The model under review builds one solid part; all positions refer to its coordinate system, in mm. A direction names the side the tool comes from. Coordinates: 2 decimals unless noted, no trailing zeros. Write each loop counter-clockwise with the first axis right and the second up, starting at its lowest first coordinate (ties: lowest second). Pieces come first, ordered by that corner, then holes. Notation, with made-up numbers: (3, -19.75) - (36, -19.75) arc R19 cw to (36, -7.75) - close; hole circle Ø1 at (46.25, 59.5). An arc over 180 degrees is marked (long way). Return JSON: item names as keys, results as strings. Group by question number.
(1) We need section C-C on z = 7.5. State the section outline as (x, y) points (3 decimals).
(2) For pin 1 Ø1.5 at (x, z) = (-7, -12.5) entering from -Y; pin 2 Ø2 at (x, y) = (-4.5, 6) entering from +Z; pin 3 Ø4.5 at (x, z) = (-1.5, 4.5) entering from +Y (3 decimals); pin 4 Ø5 at (y, z) = (-6.5, -3.5) entering from +X, all flat-tipped, find the tip position at first contact; note any pin that passes through.
(3) To check wall thickness, follow L1, parallel to Y at x = 0, z = -8.25 (3 decimals); L2, parallel to Y at x = 1.75, z = -2; L3, parallel to X at y = -4, z = 5 (3 decimals). State the ranges of each line that lie inside material, in increasing order. Write a range as from..to.
(4) Tool access review of faces 1 (the face through (10.045, 0, 7)), 2 (the face through (1, 10.06, 7)), 3 (the face through (6, 0, -25)), 4 (the face through (5.2, 1.4, -0.48)): name each direction out of +Z, -Z, +X, -X, +Y, -Y from which nothing blocks a thin tool from reaching the whole face with its end or side.
(5) We need section A-A on y = 0. State the section outline as (x, z) points (3 decimals), then the cut area to 3 significant figures.
(6) We need section D-D on z = -18. State the section outline as (x, y) points (3 decimals).
(7) Draft analysis for pull direction Y (two halves, no side actions). For faces 5 (the face through (-7, -2, 15)), 6 (the face through (-10.4, -7.974, -5.28)), 7 (the face through (1, -7.46, 7)), state which applies: released by +Y, released by -Y, zero draft, split by the parting line, or undercut.
(8) We need section B-B on x = 0. State the section outline as (y, z) points (3 decimals), then the cut area to 3 significant figures.
```python
from build123d import *

# Parameters (mm, degrees)
F1_R          = 13.105
F1_R_2        = 5
F2_DEPTH      = 25
F2_DEPTH_BACK = 15
F5_DEPTH      = 15.48


with BuildPart() as f2:
    # F1 (on Top) → F2 (new body, two sides)
    with BuildSketch(Plane.XY) as f2_sk:
        Circle(F1_R)
        Circle(F1_R_2, mode=Mode.SUBTRACT)
    extrude(amount=-F2_DEPTH)
    extrude(f2_sk.sketch, amount=F2_DEPTH_BACK)

    # F4 (on offset) → F5 (cut)
    with BuildSketch(Plane.XY.offset(15)):
        Polygon((10.0449961981, 10.0600004722), (-6.8450038019, 10.0600004722), (-6.8450038019, -5.8399995278), (-6.8450038019, -7.4599995278), (10.0449961981, -7.4599995278), align=None)
    extrude(amount=-F5_DEPTH, mode=Mode.SUBTRACT)


solid = f2.part
```
Ans:
{
 "1": {"outline": "(-6.845, -7.46) - (-6.845, 10.06) - (8.399, 10.06) arc R13.105 ccw (long way) to (10.045, 8.417) - (10.045, -7.46) - close"},
 "2": {"pin 1": "y = -11.52", "pin 2": "z = -0.48", "pin 3": "y = 13.105", "pin 4": "x = 12.48"},
 "3": {"L1": "-13.105..-5, 5..13.105", "L2": "-12.99..-4.68, 4.68..12.99", "L3": "-12.48..-6.845, 10.045..12.48"},
 "4": {"face 1": "+Z, +Y", "face 2": "+Z, +X", "face 3": "-Z, +X, -X, +Y, -Y", "face 4": "+Z"},
 "5": {"outline": "(-13.105, -25) - (-5, -25) - (-5, -0.48) - (-6.845, -0.48) - (-6.845, 15) - (-13.105, 15) - close; (5, -25) - (13.105, -25) - (13.105, 15) - (10.045, 15) - (10.045, -0.48) - (5, -0.48) - close", "area": "542 mm²"},
 "6": {"outline": "circle Ø26.21 at (0, 0); hole circle Ø10 at (0, 0)"},
 "7": {"face 5": "zero draft", "face 6": "split by the parting line", "face 7": "undercut"},
 "8": {"outline": "(-13.105, -25) - (-5, -25) - (-5, -0.48) - (-7.46, -0.48) - (-7.46, 15) - (-13.105, 15) - close; (5, -25) - (13.105, -25) - (13.105, 15) - (10.06, 15) - (10.06, -0.48) - (5, -0.48) - close", "area": "532 mm²"}
}
